The listing builds one solid part. Answer for the finished solid, in the listing's coordinates (mm). Face numbers are marked on the shaded views. A direction names the side the tool comes from. Give positions to 0.01 mm unless a question says otherwise; leave off trailing zeros. Loops run counter-clockwise (first coordinate to the right, second up) from the corner with the lowest first, then second, coordinate; pieces in that order, holes last. Notation, with made-up numbers: (-7.5, 85) - (31.5, 85) arc R11 ccw to (31.5, 90) - close; hole circle Ø4 at (77.25, 38). An arc over 180 degrees is marked (long way). Answer as CSV lines item,"result". Start each with the question number.
1) A cutting plane is placed at A-A (z = -10.5). Determine the outline of the cut face in (x, y).
2) Find the intervals of material crossed by line 1 along X through (y, z) = (1.15, -10.5); line 2 along Z through (x, y) = (7.5, 9); line 3 along Y through (x, z) = (14, -7.75), in increasing order.
3) A cutting plane is placed at B-B (x = 16). Determine the outline of the cut face in (y, z).
4) A cutting plane is placed at D-D (x = 12.25). Determine the outline of the cut face in (y, z), and give its area (4 significant figures).
5) A cutting plane is placed at C-C (y = 10.5). Determine the outline of the cut face in (x, z).
6) For the marked faces 1 and 2, determine the directions among +Z, -Z, +X, -X, +Y, -Y from which every point of the face is accessible in a straight line to the end or side of a thin tool.
7) Flat-ended cylindrical pins translate along their axes: pin 1 (4 mm diameter, centred on x = 16, z = -10.5, fed in from +Y); pin 2 (1.5 mm diameter, centred on x = 12, y = 9, fed in from -Z). Find the tip coordinate at first contact, or state that the pin passes through.
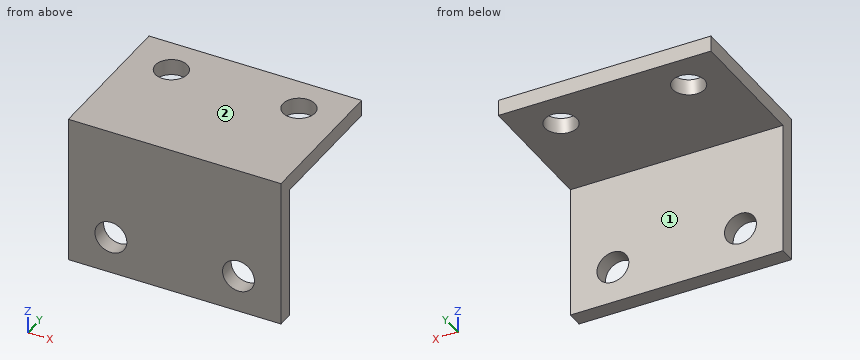
```python
from build123d import *

# Parameters (mm, degrees)
EXTRUDE_1_DEPTH     = 20
SKETCH_2_R          = 1.5
CUT_EXTRUDE_1_DEPTH = 28.427176304
SKETCH_3_R          = 1.5
CUT_EXTRUDE_2_DEPTH = 28.427176304


with BuildPart() as part:
    # 草图1 → 凸台-拉伸1 (new body)
    with BuildSketch(Plane(origin=(0, 0, 0), x_dir=(0, 0, -1), z_dir=(1, 0, 0))):
        Polygon((0, 0), (0, 14), (1.5, 14), (1.5, 1.5), (14, 1.5), (14, 0), align=None)
    extrude(amount=EXTRUDE_1_DEPTH)

    # 草图2 → 切除-拉伸1 (cut, through all)
    with BuildSketch(Plane(origin=(0, 0, -1.5), x_dir=(-1, 0, 0), z_dir=(0, 0, -1))):
        with Locations(Location((-16, 10.5, 0), (0, 0, 90))):
            Circle(SKETCH_2_R)
        with Locations(Location((-4, 10.5, 0), (0, 0, 90))):
            Circle(SKETCH_2_R)
    extrude(amount=-CUT_EXTRUDE_1_DEPTH, mode=Mode.SUBTRACT)

    # 草图3 → 切除-拉伸2 (cut, through all)
    with BuildSketch(Plane(origin=(0, 1.5, 0), x_dir=(1, 0, 0), z_dir=(0, 1, 0))):
        with Locations(Location((4, 10.5, 0), (0, 0, 270))):
            Circle(SKETCH_3_R)
        with Locations(Location((16, 10.5, 0), (0, 0, 270))):
            Circle(SKETCH_3_R)
    extrude(amount=-CUT_EXTRUDE_2_DEPTH, mode=Mode.SUBTRACT)


solid = part.part
```
Ans:
1,outline,"(0, 0) - (2.5, 0) - (2.5, 1.5) - (0, 1.5) - close; (5.5, 0) - (14.5, 0) - (14.5, 1.5) - (5.5, 1.5) - close; (17.5, 0) - (20, 0) - (20, 1.5) - (17.5, 1.5) - close"
2,line 1,"0 to 2.5, 5.5 to 14.5, 17.5 to 20"
2,line 2,"-1.5 to 0"
2,line 3,"0 to 1.5"
3,outline,"(0, -14) - (1.5, -14) - (1.5, -12) - (0, -12) - close; (0, -9) - (1.5, -9) - (1.5, -1.5) - (9, -1.5) - (9, 0) - (0, 0) - close; (12, -1.5) - (14, -1.5) - (14, 0) - (12, 0) - close"
4,outline,"(0, -14) - (1.5, -14) - (1.5, -1.5) - (14, -1.5) - (14, 0) - (0, 0) - close"
4,area,"39.75 mm2"
5,outline,"(0, -1.5) - (2.5, -1.5) - (2.5, 0) - (0, 0) - close; (5.5, -1.5) - (14.5, -1.5) - (14.5, 0) - (5.5, 0) - close; (17.5, -1.5) - (20, -1.5) - (20, 0) - (17.5, 0) - close"
6,face 1,"-Z, +X, -X, +Y"
6,face 2,"+Z, +X, -X, +Y, -Y"
7,pin 1,"y = 1.5"
7,pin 2,"z = -1.5"
